from build123d import *

# Parameters (mm, degrees)
F0_W      = 89.611202
F0_H      = 91.744802
F1_DEPTH  = 25.4
F2_R      = 20.32
F3_W      = 49.377598
F3_H      = 50.9016
F1_FACE_W = 48.971202
F1_FACE_H = 51.104802
F4_DEPTH  = 127


with BuildPart() as f1:
    # F0 (on Front) → F1 (new body)
    with BuildSketch(Plane.XZ):
        Rectangle(F0_W, F0_H)
    extrude(amount=F1_DEPTH)

    # F2
    f2_edges = [f1.edges().sort_by_distance(p)[0] for p in [
        (44.805601, -25.4, 0),
        (0, -25.4, 45.872401),
        (-44.805601, -25.4, 0),
        (0, -25.4, -45.872401),
    ]]
    fillet(f2_edges, radius=F2_R)

    # F3 (on Front) + F1_face (on face) → F4 (cut)
    with BuildSketch(Plane.XZ):
        Rectangle(F3_W, F3_H)
    with BuildSketch(Plane.XZ.offset(25.4)):
        Rectangle(F1_FACE_W, F1_FACE_H)
    extrude(amount=-F4_DEPTH, mode=Mode.SUBTRACT)


solid = f1.part
Input: part model. Units: mm. Frame: model coordinates. A direction names the side the tool comes from. Give positions to 0.01 mm unless a question says otherwise; leave off trailing zeros. Write each loop counter-clockwise with the first axis right and the second up, starting at its lowest first coordinate (ties: lowest second). Pieces come first, ordered by that corner, then holes.
Q1. Section A-A, the plane z = -3. Output: boundary loops of the cut face in (x, y), plus the area to 3 significant figures.
Q2. Set-up query: faces 4 (the face through (24.486, -13, 0)), 5 (the face through (0.63, -19.29, -40.08)). Return all of +Z, -Z, +X, -X, +Y, -Y with unobstructed straight access to the full face (end or side cutting, diameter ignored); none if empty.
Q3. Pull-direction query (X, two-part tool) for faces 1 (the face through (0, -13, -25.552)), 2 (the face through (0.63, -19.29, 40.08)), 3 (the face through (-39, -19.3, 0.6)); classes: pulls with the +X half, pulls with the -X half, needs draft (parallel to the pull), parting line crosses it, or undercut.
Q4. Section D-D, the plane y = -8. Output: boundary loops of the cut face in (x, z).
Q5. Material intervals for probe 1 along X at (y, z) = (-3, 10.5); probe 2 along X at (y, z) = (-18.5, 3.5); probe 3 along Z at (x, y) = (19, -21.75), sorted ascending.
Q6. Section B-B, the plane x = 9. Output: boundary loops of the cut face in (y, z), plus the area to 3 significant figures.
Q7. First-contact query: P1, Ø6, axis at y = -16, z = 31, coming from the -X side; P2, Ø8, axis at y = -15.5, z = 6, coming from the -X side; P3, Ø1.5, axis at x = -28.5, y = -22.5, coming from the -Z side. Flat tips, straight axial feed; report the tip coordinate or a pass-through.
Q8. Section C-C, the plane y = -14.25. Output: boundary loops of the cut face in (x, z), plus the area to 3 significant figures.
Filled in:
1. outline: (-44.81, -5.08) arc R20.32 ccw to (-24.49, -25.4) - (-24.49, 0) - (-44.81, 0) - close; (24.49, -25.4) arc R20.32 ccw to (44.81, -5.08) - (44.81, 0) - (24.49, 0) - close
1. area: 855 mm2
2. face 4: +Y, -Y
2. face 5: -Z, +X, -X, -Y
3. face 1: undercut
3. face 2: needs draft
3. face 3: pulls with the -X half
4. outline: (-44.59, -45.66) - (44.59, -45.66) - (44.59, 45.66) - (-44.59, 45.66) - close; hole (-24.49, -25.55) - (24.49, -25.55) - (24.49, 25.55) - (-24.49, 25.55) - close
5. probe 1: x = -44.81 to -24.49, 24.49 to 44.81
5. probe 2: x = -39.74 to -24.49, 24.49 to 39.74
5. probe 3: z = -37.17 to -25.55, 25.55 to 37.17
6. outline: (-25.4, -25.55) arc R20.32 ccw to (-5.08, -45.87) - (0, -45.87) - (0, -25.55) - close; (-25.4, 25.55) - (0, 25.55) - (0, 45.87) - (-5.08, 45.87) arc R20.32 ccw to start
6. area: 855 mm2
7. P1: stops at x = -43.2
7. P2: stops at x = -43.76
7. P3: stops at z = -37.17
8. outline: (-42.62, -43.69) - (42.62, -43.69) - (42.62, 43.69) - (-42.62, 43.69) - close; hole (-24.49, -25.55) - (24.49, -25.55) - (24.49, 25.55) - (-24.49, 25.55) - close
8. area: 4,940 mm2
